Check sheet for the modelled part. Datum: model origin and axes. Units: mm. Give positions to 0.01 mm unless a question says otherwise; leave off trailing zeros. Loops run counter-clockwise (first coordinate to the right, second up) from the corner with the lowest first, then second, coordinate; pieces in that order, holes last. Notation, with made-up numbers: (60, 28.25) - (112, 28.25) arc R20 cw to (112, 32.25) - close; hole circle Ø4 at (-32, 0). An arc over 180 degrees is marked (long way). Use one line per item in the form item = value.
from build123d import *

# Parameters (mm, degrees)
SKETCH1_R           = 2.4
BOSS_EXTRUDE2_DEPTH = 3


with BuildPart() as part:
    # Sketch1 → Boss-Extrude2 (new body)
    with BuildSketch(Plane(origin=(0, 0, 0), x_dir=(1, 0, 0), z_dir=(0, 1, 0))):
        with BuildLine():
            Line((16.145, 4.035), (-16.145, 4.035))
            ThreePointArc((-16.145, 4.035), (-18.99817587, 2.853175854), (-20.18, -2.2e-08))
            ThreePointArc((-20.18, -2.2e-08), (-18.998175854, -2.85317587), (-16.145, -4.035))
            Line((-16.145, -4.035), (16.145, -4.035))
            ThreePointArc((16.145, -4.035), (18.998175862, -2.853175862), (20.18, 0))
            ThreePointArc((20.18, 0), (18.998175862, 2.853175862), (16.145, 4.035))
        make_face()
        with Locations(Location((-16.145, 0, 0), (0, 0, 270))):
            Circle(SKETCH1_R, mode=Mode.SUBTRACT)
        with Locations(Location((0, 0, 0), (0, 0, 270))):
            Circle(SKETCH1_R, mode=Mode.SUBTRACT)
        with Locations(Location((16.145, 0, 0), (0, 0, 270))):
            Circle(SKETCH1_R, mode=Mode.SUBTRACT)
    extrude(amount=BOSS_EXTRUDE2_DEPTH)


solid = part.part
Item 1: Section check A-A on x = 0. Record the boundary of the cut face in (y, z) (3 decimals).
Answer block:
outline = (0, -4.035) - (3, -4.035) - (3, -2.4) - (0, -2.4) - close; (0, 2.4) - (3, 2.4) - (3, 4.035) - (0, 4.035) - close
Item 2: Section check C-C on z = -2. Record the boundary of the cut face in (x, y), then the cut area to 3 significant figures.
Answer block:
outline = (-19.65, 0) - (-17.47, 0) - (-17.47, 3) - (-19.65, 3) - close; (-14.82, 0) - (-1.33, 0) - (-1.33, 3) - (-14.82, 3) - close; (1.33, 0) - (14.82, 0) - (14.82, 3) - (1.33, 3) - close; (17.47, 0) - (19.65, 0) - (19.65, 3) - (17.47, 3) - close
area = 94.0 mm2
Item 3: Section check B-B on y = 1.7. Record the boundary of the cut face in (x, z) (3 decimals), then the cut area to 3 significant figures.
Answer block:
outline = (-16.145, -4.035) - (16.145, -4.035) arc R4.035 ccw to (16.145, 4.035) - (-16.145, 4.035) arc R4.035 ccw to start; hole circle Ø4.8 at (-16.145, 0); hole circle Ø4.8 at (0, 0); hole circle Ø4.8 at (16.145, 0)
area = 257 mm2
Item 4: Mould release check, pull along X, two halves, no side actions. Record for faces 1 (the face through (0, 1, 4.035)), 2 (the face through (13.8, 1.48, -0.52)): released by +X, released by -X, zero draft, split by the parting line, or undercut.
Answer block:
face_1 = zero draft
face_2 = undercut
Item 5: Thickness scan on L1, parallel to X at y = 0.45, z = 1.25; L2, parallel to X at y = 2.65, z = 0.25; L3, parallel to Z at x = -1.5, y = 2.2 (1 decimal). Record the ranges inside material, lowest first.
Answer block:
L1 = -19.98 to -18.19, -14.1 to -2.05, 2.05 to 14.1, 18.19 to 19.98
L2 = -20.17 to -18.53, -13.76 to -2.39, 2.39 to 13.76, 18.53 to 20.17
L3 = -4 to -1.9, 1.9 to 4
